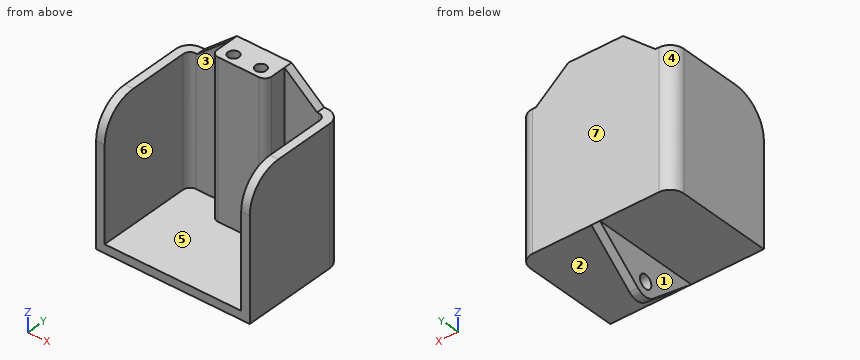
from build123d import *

# Parameters (mm, degrees)
SKETCH1_R           = 4
BOSS_EXTRUDE1_DEPTH = 120
CUT_EXTRUDE2_DEPTH  = 169.5
SKETCH4_R           = 5
BOSS_EXTRUDE3_DEPTH = 3.125
BOSS_EXTRUDE5_REACH = 156.803
SKETCH6_W           = 106.515256917
SKETCH6_H           = 6.25
FILLET1_R           = 25


with BuildPart() as part:
    # Sketch1 → Boss-Extrude1 (new body)
    with BuildSketch(Plane.XY):
        with BuildLine():
            Line((-45, 53.75), (-20, 53.75))
            Line((-20, 53.75), (-20, 42.5))
            ThreePointArc((-20, 42.5), (-18.535533906, 38.964466094), (-15, 37.5))
            Line((-15, 37.5), (15, 37.5))
            ThreePointArc((15, 37.5), (18.535533906, 38.964466094), (20, 42.5))
            Line((20, 42.5), (20, 53.75))
            Line((20, 53.75), (45, 53.75))
            ThreePointArc((45, 53.75), (48.535533906, 52.285533906), (50, 48.75))
            Line((50, 48.75), (50, -20))
            Line((50, -20), (56.25, -20))
            Line((56.25, -20), (56.25, 50))
            ThreePointArc((56.25, 50), (53.321067812, 57.071067812), (46.25, 60))
            Line((46.25, 60), (-46.25, 60))
            ThreePointArc((-46.25, 60), (-53.321067812, 57.071067812), (-56.25, 50))
            Line((-56.25, 50), (-56.25, -20))
            Line((-56.25, -20), (-50, -20))
            Line((-50, -20), (-50, 48.75))
            ThreePointArc((-50, 48.75), (-48.535533906, 52.285533906), (-45, 53.75))
        make_face()
        with Locations((-10, 45)):
            Circle(SKETCH1_R, mode=Mode.SUBTRACT)
        with Locations(Location((10, 45, 0), (0, 0, 180))):
            Circle(SKETCH1_R, mode=Mode.SUBTRACT)
    extrude(amount=BOSS_EXTRUDE1_DEPTH)

    # Sketch2 → Cut-Extrude2 (cut, symmetric)
    with BuildSketch(Plane(origin=(0, 0, 0), x_dir=(1, 0, 0), z_dir=(0, 1, 0))):
        Polygon((-20, -120), (-43.835071852, -100), (-56.25, -100), (-56.25, -170), (56.25, -170), (56.25, -100), (43.835071852, -100), (20, -120), align=None)
    extrude(amount=CUT_EXTRUDE2_DEPTH, both=True, mode=Mode.SUBTRACT)

    # Sketch4 → Boss-Extrude3 (add, symmetric)
    with BuildSketch(Plane(origin=(0, 0, 0), x_dir=(0, 0, -1), z_dir=(1, 0, 0))):
        with BuildLine():
            Line((0, 60), (0, -20))
            Line((0, -20), (28, 13.266499161))
            ThreePointArc((28, 13.266499161), (30.456578482, 20), (28, 26.733500839))
            Line((28, 26.733500839), (0, 60))
        make_face()
        with Locations((20, 20)):
            Circle(SKETCH4_R, mode=Mode.SUBTRACT)
    extrude(amount=BOSS_EXTRUDE3_DEPTH, both=True)

    # Boss-Extrude5: up to this face of the body (flat: up to its plane)
    boss_extrude5_end = Plane(part.part.faces().sort_by_distance((-32.103527113, 53.75, 54.932363347))[0])
    # Sketch6 → Boss-Extrude5 (add, up to the picked face)
    with BuildSketch(Plane.XZ.offset(20), mode=Mode.PRIVATE) as boss_extrude5_sk1:
        with Locations((-0.086289354, 3.125)):
            Rectangle(SKETCH6_W, SKETCH6_H)
    boss_extrude5_tool1 = split(extrude(boss_extrude5_sk1.sketch, amount=-BOSS_EXTRUDE5_REACH, mode=Mode.PRIVATE), bisect_by=boss_extrude5_end, keep=Keep.BOTH, mode=Mode.PRIVATE)
    add(boss_extrude5_tool1.solids().sort_by(Axis((-0.086289, -20, 3.125), (0, 1, 0)))[0])

    # Fillet1
    fillet1_edges = [part.edges().sort_by_distance(p)[0] for p in [
        (53.125, -20, 100),
        (-53.125, -20, 100),
    ]]
    fillet(fillet1_edges, radius=FILLET1_R)


solid = part.part
Model file for the job. Use its own axes, mm. Face numbers are marked on the shaded views. A direction names the side the tool comes from. Coordinates: 2 decimals unless noted, no trailing zeros. Order: outer loops, then holes, each group sorted by start corner. A loop starts at its lowest first (then second) coordinate and runs counter-clockwise, first axis right, second up. Notation, with made-up numbers: M 89.25,84 L 117.25,84 A16 ccw 117.25,106 Z; hole C 82.5,63 d6. An arc over 180 degrees is marked long. Return JSON: item names as keys, results as strings.
1. Saw through at C-C (y = 34.5). Give the cut face in (x, z) (3 decimals), and give its area (3 significant figures).
Ans:
{"outline": "M -56.25,0 L -3.125,0 L -3.125,-21.463 L 3.125,-21.463 L 3.125,0 L 56.25,0 L 56.25,100 L 50,100 L 50,6.25 L -50,6.25 L -50,100 L -56.25,100 Z", "area": "2,010 mm^2"}
2. Tool access for the marked faces 1, 2 and 3: list every direction of +Z, -Z, +X, -X, +Y, -Y with a clear straight run to the whole face (end or side of a thin tool).
Ans:
{"face 1": "-Z, -X, +Y, -Y", "face 2": "-Z, +X, +Y, -Y", "face 3": "+Z, -Y"}
3. Saw through at B-B (x = -10). Give the cut face in (y, z).
Ans:
{"outline": "M -20,0 L 60,0 L 60,120 L 49,120 L 49,6.25 L 41,6.25 L 41,120 L 37.5,120 L 37.5,6.25 L -20,6.25 Z"}
4. Drill centre lines: probe 1 along X at (y, z) = (45, 81); probe 2 along X at (y, z) = (-5.5, 88); probe 3 along Y at (x, z) = (10, 49). Where is each one in solid material? Low to high.
Ans:
{"probe 1": "-56.25 to -50, -20 to -14, -6 to 6, 14 to 20, 50 to 56.25", "probe 2": "-56.25 to -50, 50 to 56.25", "probe 3": "37.5 to 41, 49 to 60"}
5. Pull direction X, two halves, no side cores. Call the marked faces 4, 5, 6 and 7: +X half, -X half, draft (parallel to the pull), parting line (faces both ways), or undercut.
Ans:
{"face 4": "-X half", "face 5": "undercut", "face 6": "undercut", "face 7": "draft"}
6. Flat gauge pins, fed straight in: pin 1 (11.5 mm diameter, centred on y = 20, z = -20, fed in from +X) (3 decimals); pin 2 (8 mm diameter, centred on x = 30.5, y = 40.5, fed in from +Z); pin 3 (1.5 mm diameter, centred on y = 1.5, z = -7, fed in from -X) (3 decimals). Where does each tip first touch, or does it go through?
Ans:
{"pin 1": "x = 3.125", "pin 2": "z = 6.25", "pin 3": "x = -3.125"}
7. Saw through at D-D (z = -20). Give the cut face in (x, y) (3 decimals).
Ans:
{"outline": "M -3.125,3.762 L 3.125,3.762 L 3.125,15 L -3.125,15 Z; M -3.125,25 L 3.125,25 L 3.125,36.238 L -3.125,36.238 Z"}
8. Saw through at A-A (z = 9). Give the cut face in (x, y).
Ans:
{"outline": "M -56.25,-20 L -50,-20 L -50,48.75 A5 cw -45,53.75 L -20,53.75 L -20,42.5 A5 ccw -15,37.5 L 15,37.5 A5 ccw 20,42.5 L 20,53.75 L 45,53.75 A5 cw 50,48.75 L 50,-20 L 56.25,-20 L 56.25,50 A10 ccw 46.25,60 L -46.25,60 A10 ccw -56.25,50 Z; hole C -10,45 d8; hole C 10,45 d8"}
